Build history of the part. All positions in model axes, mm. Face numbers are marked on the shaded views. A direction names the side the tool comes from. Give positions to 0.01 mm unless a question says otherwise; leave off trailing zeros. Loops run counter-clockwise (first coordinate to the right, second up) from the corner with the lowest first, then second, coordinate; pieces in that order, holes last. Notation, with made-up numbers: M -7,48 L 15,48 A7 cw 15,54 Z; hole C 68.25,73 d9. An arc over 180 degrees is marked long. Put each result on its own line as item: value.
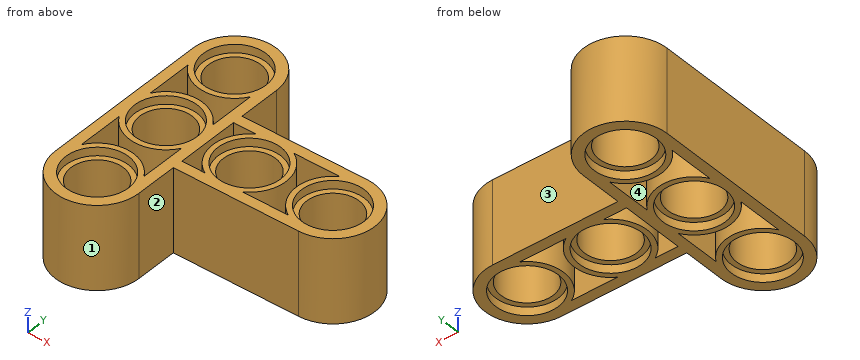
Autodesk Inventor part; units mm, degrees
ref_plane "YZ Plane" through (0, 0, 0) normal (1, 0, 0) x (0, 1, 0)
ref_plane "XZ Plane" through (0, 0, 0) normal (0, 1, 0) x (-1, 0, 0)
ref_plane "XY Plane" through (0, 0, 0) normal (0, 0, 1) x (1, 0, 0)
sketch "Sketch1" plane through (0, 0, 0) normal (0, 0, 1) x (1, 0, 0)
  arc A0 (0, -4) -> (0, 4) centre (0, 0) ccw
  arc A1 (-12, 8) -> (-20, 8) centre (-16, 8) ccw
  arc A2 (-20, -8) -> (-12, -8) centre (-16, -8) ccw
  line L0 (-20, -8) -> (-20, 8)
  line L1 (0, 4) -> (-12, 4)
  line L2 (0, -4) -> (-12, -4)
  line L3 (-12, 8) -> (-12, 4)
  line L4 (-12, -4) -> (-12, -8)
  line L5 (-24.8, 0) -> (8.8, 0)
  line L6 (0, -16.8) -> (0, 16.8)
  dimension "d3" = 4
  dimension "d4" = 4
  dimension "d5" = 4
  dimension "d6" = 16
  dimension "d8" = 8
  dimension "d10" = 16
  dimension "d11" = 0
  dimension "d12" = 0
  dimension "d13" = 4
extrude "Extrusion1" add sketch "Sketch1" along normal blind 8
sketch "Sketch3" plane through (0, 0, 8) normal (0, 0, 1) x (1, 0, 0)
  arc A0 (0, -4) -> (0, 4) centre (0, 0) ccw
  circle A1 centre (0, 0) radius 2.5
  line L0 (-24.8, 0) -> (8.8, 0)
  circle A2 centre (-8, 0) radius 2.5
  dimension "d24" = 5
  dimension "d30" = 8
extrude "Extrusion2" cut sketch "Sketch3" against normal through all
sketch "Sketch4" plane through (0, 0, 8) normal (0, 0, 1) x (1, 0, 0)
  arc A0 (-20, -8) -> (-12, -8) centre (-16, -8) ccw
  circle A1 centre (-16, -8) radius 2.5
  line L0 (0, -16.8) -> (0, 16.8)
  circle A2 centre (-16, 0) radius 2.5
  circle A3 centre (-16, 8) radius 2.5
  dimension "d34" = 5
  dimension "d40" = 8
extrude "Extrusion3" cut sketch "Sketch4" against normal through all
sketch "Sketch5" plane through (0, 0, 8) normal (0, 0, 1) x (1, 0, 0)
  circle A0 centre (-16, 8) radius 2.5
  circle A1 centre (-16, 0) radius 2.5
  circle A2 centre (-16, -8) radius 2.5
  circle A3 centre (-8, 0) radius 2.5
  circle A4 centre (0, 0) radius 2.5
  arc A5 (-20, -8) -> (-12, -8) centre (-16, -8) ccw
  arc A6 (0, -4) -> (0, 4) centre (0, 0) ccw
  arc A7 (-12, 8) -> (-20, 8) centre (-16, 8) ccw
  circle A8 centre (-16, -8) radius 3
  circle A9 centre (-16, 0) radius 3
  circle A10 centre (-16, 8) radius 3
  circle A11 centre (-8, 0) radius 3
  circle A12 centre (0, 0) radius 3
  dimension "d44" = 6
  dimension "d45" = 6
  dimension "d46" = 6
  dimension "d47" = 6
  dimension "d48" = 6
extrude "Extrusion4" cut sketch "Sketch5" against normal blind 0.8
sketch "Sketch6" plane through (0, 0, 0) normal (0, 0, -1) x (-1, 0, 0)
  circle A0 centre (16, 8) radius 2.5
  circle A1 centre (16, 0) radius 2.5
  circle A2 centre (16, -8) radius 2.5
  circle A3 centre (8, 0) radius 2.5
  circle A4 centre (0, 0) radius 2.5
  arc A5 (12, -8) -> (20, -8) centre (16, -8) ccw
  arc A6 (20, 8) -> (12, 8) centre (16, 8) ccw
  arc A7 (0, 4) -> (0, -4) centre (0, 0) ccw
  circle A8 centre (8, 0) radius 3
  circle A9 centre (16, 8) radius 3
  circle A10 centre (0, 0) radius 3
  circle A11 centre (16, 0) radius 3
  circle A12 centre (16, -8) radius 3
  dimension "d52" = 6
  dimension "d53" = 6
  dimension "d54" = 6
  dimension "d55" = 6
  dimension "d56" = 6
extrude "Extrusion5" cut sketch "Sketch6" against normal blind 0.8
sketch "Sketch7" plane through (0, 0, 8) normal (0, 0, 1) x (1, 0, 0)
  circle A0 centre (-16, -8) radius 3
  circle A1 centre (-16, 0) radius 3
  arc A2 (-20, -8) -> (-12, -8) centre (-16, -8) ccw
  arc A3 (-13, -6.1972) -> (-19, -6.1972) centre (-16, -8) ccw
  line L0 (-19, -1.8028) -> (-19, -6.1972)
  line L1 (-13, -1.8028) -> (-13, -6.1972)
  arc A4 (-19, -1.8028) -> (-13, -1.8028) centre (-16, 0) ccw
  line L2 (0, -16.8) -> (0, 16.8)
  arc A5 (-13, 1.8028) -> (-19, 1.8028) centre (-16, 0) ccw
  line L3 (-19, 6.1972) -> (-19, 1.8028)
  line L4 (-13, 6.1972) -> (-13, 1.8028)
  arc A6 (-19, 6.1972) -> (-13, 6.1972) centre (-16, 8) ccw
  dimension "d59" = 3.5
  dimension "d60" = 3.5
  dimension "d66" = 8
extrude "Extrusion6" cut sketch "Sketch7" against normal through all contours A3 L0 A4 L1 | A5 L3 A6 L4
sketch "Sketch8" plane through (0, 0, 8) normal (0, 0, 1) x (1, 0, 0)
  line L0 (-13, -1.8028) -> (-13, -6.1972)
  circle A0 centre (-16, 0) radius 3
  circle A1 centre (-8, 0) radius 3
  arc A2 (0, -4) -> (0, 4) centre (0, 0) ccw
  line L1 (-12, 4) -> (0, 4)
  line L2 (-12, 8) -> (-12, 4)
  arc A3 (-1.8028, 3) -> (-1.8028, -3) centre (0, 0) ccw
  line L3 (-12, 3) -> (-12, -3)
  line L4 (-6.1972, -3) -> (-1.8028, -3)
  line L5 (-6.1972, 3) -> (-1.8028, 3)
  arc A4 (-9.8028, 3) -> (-9.8028, -3) centre (-8, 0) ccw
  arc A5 (-6.1972, -3) -> (-6.1972, 3) centre (-8, 0) ccw
  line L6 (-9.8028, 3) -> (-12, 3)
  line L7 (-9.8028, -3) -> (-12, -3)
  dimension "d72" = 3.5
  dimension "d73" = 3.5
  dimension "d74" = 3.5
  dimension "d75" = 2.1972
extrude "Extrusion7" cut sketch "Sketch8" against normal through all contours A3 L4 A5 L5 | L6 A4 L7 L3
properties part number "5TM Beam"
Q1. Slice it at B-B (x = -8). List the corners of the cut face in (y, z).
Here are the results:
outline: M -4,0 L -3,0 L -3,0.8 L -2.5,0.8 L -2.5,7.2 L -3,7.2 L -3,8 L -4,8 Z; M 2.5,0.8 L 3,0.8 L 3,0 L 4,0 L 4,8 L 3,8 L 3,7.2 L 2.5,7.2 Z
Q2. Slice it at C-C (y = 8.75). List the corners of the cut face in (x, z).
Here are the results:
outline: M -19.93,0 L -18.9,0 L -18.9,0.8 L -18.38,0.8 L -18.38,7.2 L -18.9,7.2 L -18.9,8 L -19.93,8 Z; M -13.62,0.8 L -13.1,0.8 L -13.1,0 L -12.07,0 L -12.07,8 L -13.1,8 L -13.1,7.2 L -13.62,7.2 Z
Q3. Probe line 1 (Y direction, x = -16, z = 7.45); line 2 (Y direction, x = -8, z = 4.25); line 3 (X direction, y = -0.5, z = 3.25). List the from-to ranges inside material, lowest first. Write a range as from..to.
Here are the results:
line 1: -12..-11, -5..-4.5, -3.5..-3, 3..3.5, 4.5..5, 11..12
line 2: -4..-2.5, 2.5..4
line 3: -20..-18.45, -13.55..-12, -11.46..-10.45, -5.55..-4.54, -3.46..-2.45, 2.45..3.97
Q4. Drop flat-ended pins along their axis: pin 1 Ø3 at (x, y) = (-16.5, 7.5) entering from -Z; pin 2 Ø1.8 at (y, z) = (-1.5, 3.5) entering from +X; pin 3 Ø1 at (x, z) = (-1.5, 1) entering from -Y; pin 4 Ø3 at (x, y) = (-15, 0.5) entering from -Z. Give the stop position or say it passes through.
Here are the results:
pin 1: through
pin 2: x = 3.95
pin 3: y = -4
pin 4: z = 0.8
Q5. Tool access for the marked faces 1, 2, 3 and 4: list every direction of +Z, -Z, +X, -X, +Y, -Y with a clear straight run to the whole face (end or side of a thin tool).
Here are the results:
face 1: +Z, -Z, -Y
face 2: +Z, -Z, +X, -Y
face 3: +Z, -Z, +X, +Y
face 4: +Z, -Z
Q6. Slice it at A-A (z = 6.5). State how many separate pieces and enclosed holes the cut face has, and give its area (3 significant figures).
Here are the results:
separate pieces: 1
enclosed holes: 9
area: 159 mm²
